Autodesk Inventor part; units mm, degrees
ref_plane "YZ Plane" through (0, 0, 0) normal (1, 0, 0) x (0, 1, 0)
ref_plane "XZ Plane" through (0, 0, 0) normal (0, 1, 0) x (-1, 0, 0)
sketch "Sketch1" plane through (0, 0, 0) normal (0, 0, 1) x (1, 0, 0)
  circle A0 centre (0, 0) radius 14
  line L0 (0, 0) -> (-48, 0) construction
  circle A1 centre (-48, 0) radius 9
  line L1 (-48.9375, 8.951) -> (-1.4583, 13.9238)
  line L2 (-48.9375, -8.951) -> (-1.4583, -13.9238)
  dimension "d0" = 18
  dimension "d1" = 28
  dimension "d2" = 48
extrude "Extrusion1" add sketch "Sketch1" along normal mid plane 5
sketch "Sketch2" plane through (0, 0, 2.5) normal (0, 0, 1) x (1, 0, 0)
  arc A0 (-1.4583, -13.9238) -> (-1.4583, 13.9238) centre (0, 0) ccw
hole "Hole1" at (0, 0, 2.5) direction (0, 0, -1) diameter 15.84 end through all
sketch "Sketch3" plane through (0, 0, 2.5) normal (0, 0, 1) x (1, 0, 0)
  arc A0 (-48.9375, 8.951) -> (-48.9375, -8.951) centre (-48, 0) ccw
hole "Hole2" at (-48, 0, 2.5) direction (0, 0, -1) diameter 9 end through all
properties part number "313-01-03" material "Steel"
CAD build for the part. Positions are in the model's coordinates, mm. Round coordinates to 2 decimals unless told otherwise and drop trailing zeros. Write each loop counter-clockwise with the first axis right and the second up, starting at its lowest first coordinate (ties: lowest second). Pieces come first, ordered by that corner, then holes. Notation, with made-up numbers: M 46.5,-3.5 L 72.5,-3.5 A16 cw 72.5,14.5 Z; hole C 40.5,-2 d8. An arc over 180 degrees is marked long. Put each result on its own line as item: value. Start each with the question number.
1) Saw through at D-D, the plane z = 0.15. Write the cut outline in (x, y), and give its area (3 significant figures).
2) Pull direction Y, two halves, no side cores. Call faces 1 (the flat face through (-25.53, 11.403, -0.035)), 2 (the cylindrical face through (7.73, 1.72, -0.04)), 3 (the cylindrical face through (14, 0, 0)): pulls with the +Y half, pulls with the -Y half, needs draft (parallel to the pull), parting line crosses it, or undercut.
3) Saw through at A-A, the plane x = 0. Write the cut outline in (y, z).
4) Pin check, flat tip, straight feed: pin 1 Ø7 at (x, y) = (-48, 0) entering from -Z (3 decimals). Stop position of the tip, or through.
5) Drill centre lines: probe 1 along X at (y, z) = (0, -1.2); probe 2 along Y at (x, z) = (0, -0.9); probe 3 along Y at (x, z) = (-48, 0.6). Where is each one in solid material? Low to high. Write a range as [from, to].
6) Saw through at B-B, the plane y = 0. Write the cut outline in (x, z), and give its area (3 significant figures).
7) Saw through at C-C, the plane y = 7. Write the cut outline in (x, z).
Resolved:
1. outline: M -48.94,-8.95 L -1.46,-13.92 A14 ccw long -1.46,13.92 L -48.94,8.95 A9 ccw Z; hole C -48,0 d9; hole C 0,0 d15.84
1. area: 1,280 mm²
2. face 1: pulls with the +Y half
2. face 2: undercut
2. face 3: parting line crosses it
3. outline: M -14,-2.5 L -7.92,-2.5 L -7.92,2.5 L -14,2.5 Z; M 7.92,-2.5 L 14,-2.5 L 14,2.5 L 7.92,2.5 Z
4. pin 1: through
5. probe 1: [-57, -52.5], [-43.5, -7.92], [7.92, 14]
5. probe 2: [-14, -7.92], [7.92, 14]
5. probe 3: [-9.05, -4.5], [4.5, 9.05]
6. outline: M -57,-2.5 L -52.5,-2.5 L -52.5,2.5 L -57,2.5 Z; M -43.5,-2.5 L -7.92,-2.5 L -7.92,2.5 L -43.5,2.5 Z; M 7.92,-2.5 L 14,-2.5 L 14,2.5 L 7.92,2.5 Z
6. area: 231 mm²
7. outline: M -53.66,-2.5 L -3.7,-2.5 L -3.7,2.5 L -53.66,2.5 Z; M 3.7,-2.5 L 12.12,-2.5 L 12.12,2.5 L 3.7,2.5 Z
